Input: dimensioned drawing with shaded views. Units: mm. Origin: part minimum x, y, z. Round coordinates to 2 decimals unless told otherwise and drop trailing zeros. Loops run counter-clockwise (first coordinate to the right, second up) from the corner with the lowest first, then second, coordinate; pieces in that order, holes last. Notation, with made-up numbers: M 46,-7.75 L 104,-7.75 A27 cw 104,31.25 Z; hole C -37,-35 d1. An arc over 180 degrees is marked long. Use one line per item in the form item = value. Start each with the question number.
Q1. Section query A-A, the plane y = 69. Output: boundary loops of the cut face in (x, z) (1 decimal).
Q2. Ray query, line 1 along Y through (x, z) = (19.5, 291) (1 decimal); line 2 along Y through (x, z) = (7.25, 268.5) (1 decimal); line 3 along Z through (x, y) = (13.5, 189) (1 decimal). Return the intervals inside material, ascending.
Q3. Section query C-C, the plane x = 9.75. Output: boundary loops of the cut face in (y, z).
Q4. First-contact query: P1, Ø2, axis at x = 16, y = 127.5, coming from the -Z side; P2, Ø1, axis at x = 12.5, y = 163, coming from the +Z side (1 decimal); P3, Ø5, axis at x = 4.5, y = 283.5, coming from the +Z side; P4, Ø12, axis at x = 21.5, y = 363, coming from the +Z side. Flat tips, straight axial feed; report the tip coordinate or a pass-through.
Q5. Section query B-B, the plane z = 174.5. Output: boundary loops of the cut face in (x, y), and give its area (3 significant figures).
Q6. Section query D-D, the plane z = 559. Output: boundary loops of the cut face in (x, y).
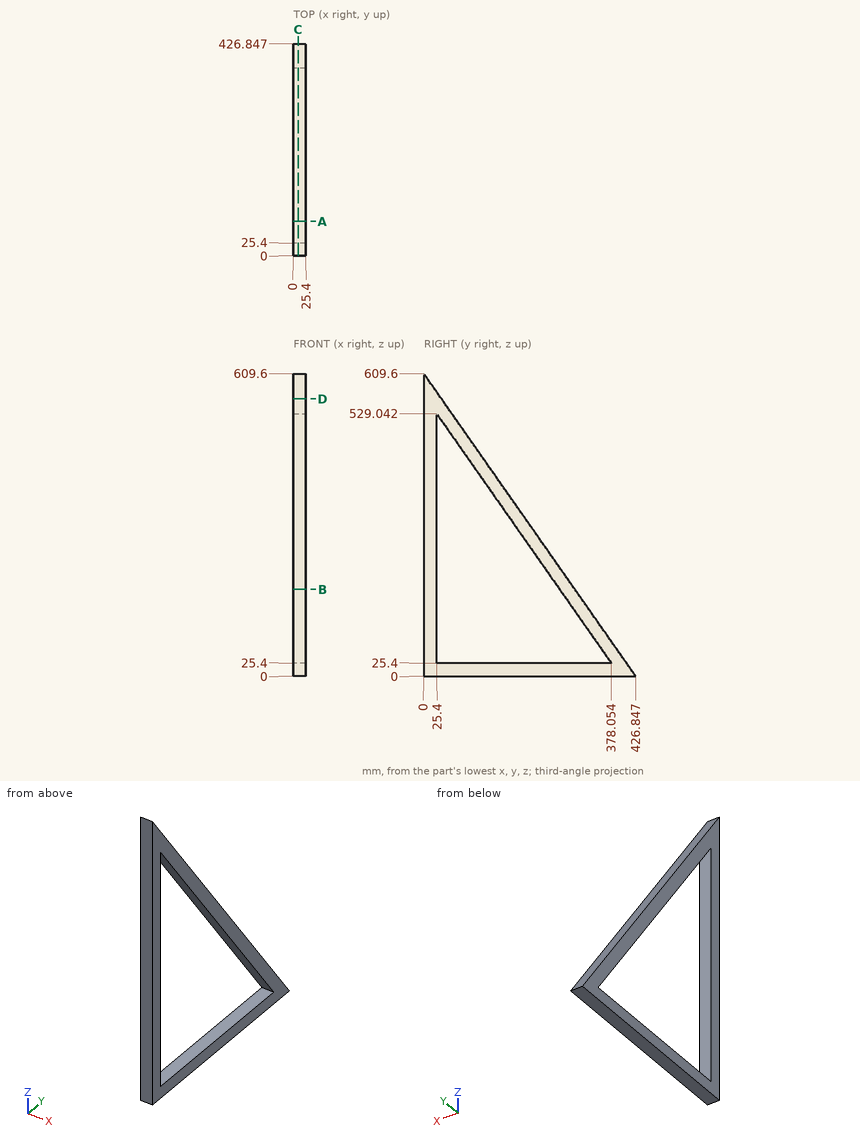
Results found:
q1.outline = M 0,0 L 25.4,0 L 25.4,25.4 L 0,25.4 Z; M 0,466.8 L 25.4,466.8 L 25.4,511.1 L 0,511.1 Z
q2.line_1 = 0 to 25.4, 192.1 to 223.1
q2.line_2 = 0 to 25.4, 207.8 to 238.8
q2.line_3 = 0 to 25.4, 295.4 to 339.7
q3.outline = M 0,0 L 426.85,0 L 0,609.6 Z; hole M 25.4,25.4 L 378.05,25.4 L 25.4,529.04 Z
q4.P1 = 0
q4.P2 = 377.5
q4.P3 = 208.29
q4.P4 = 99.75
q5.outline = M 0,0 L 25.4,0 L 25.4,25.4 L 0,25.4 Z; M 0,273.65 L 25.4,273.65 L 25.4,304.66 L 0,304.66 Z
q5.area = 1,430 mm²
q6.outline = M 0,0 L 25.4,0 L 25.4,35.43 L 0,35.43 Z
